Geometry check sheet. Reference: the model listing, model coordinates, mm. Face numbers are marked on the shaded views. A direction names the side the tool comes from. Coordinates: 2 decimals unless noted, no trailing zeros. Write each loop counter-clockwise with the first axis right and the second up, starting at its lowest first coordinate (ties: lowest second). Pieces come first, ordered by that corner, then holes.
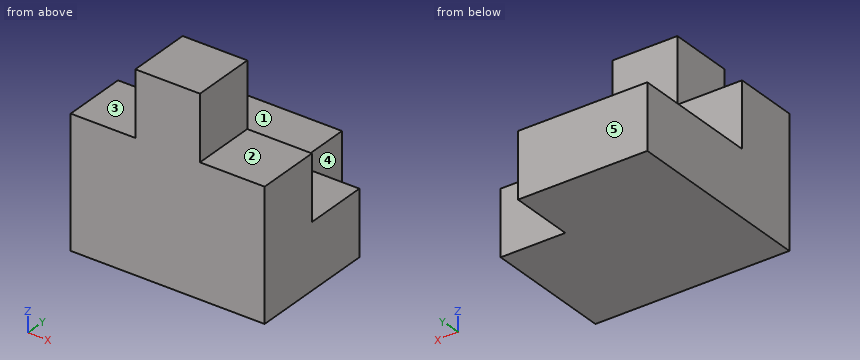
from build123d import *

# Parameters (mm, degrees)
ESBO_O2_W                = 60
ESBO_O2_H                = 20
RESSALTO_EXTRUS_O1_DEPTH = 40
ESBO_O4_W                = 20
ESBO_O4_H                = 20
CORTE_EXTRUS_O1_DEPTH    = 40
ESBO_O5_W                = 20
ESBO_O5_H                = 20
CORTE_EXTRUS_O2_DEPTH    = 40
ESBO_O7_W                = 60
ESBO_O7_H                = 40.049473908
RESSALTO_EXTRUS_O2_DEPTH = 20
ESBO_O8_W                = 40
ESBO_O8_H                = 20
RESSALTO_EXTRUS_O3_DEPTH = 20


with BuildPart() as part:
    # Esboço2 → Ressalto-extrusão1 (new body)
    with BuildSketch(Plane.XY):
        with Locations((30, 10)):
            Rectangle(ESBO_O2_W, ESBO_O2_H)
    extrude(amount=RESSALTO_EXTRUS_O1_DEPTH)

    # Esboço4 → Corte-extrusão1 (cut)
    with BuildSketch(Plane(origin=(0, 20, 0), x_dir=(1, 0, 0), z_dir=(0, 1, 0))):
        with Locations((10, -30)):
            Rectangle(ESBO_O4_W, ESBO_O4_H)
    extrude(amount=-CORTE_EXTRUS_O1_DEPTH, mode=Mode.SUBTRACT)

    # Esboço5 → Corte-extrusão2 (cut)
    with BuildSketch(Plane(origin=(0, 20, 0), x_dir=(1, 0, 0), z_dir=(0, 1, 0))):
        with Locations((50, -30)):
            Rectangle(ESBO_O5_W, ESBO_O5_H)
    extrude(amount=-CORTE_EXTRUS_O2_DEPTH, mode=Mode.SUBTRACT)

    # Esboço7 → Ressalto-extrusão2 (add)
    with BuildSketch(Plane(origin=(0, 0, 0), x_dir=(-1, 0, 0), z_dir=(0, 0, -1))):
        with Locations((-30, 20.024736954)):
            Rectangle(ESBO_O7_W, ESBO_O7_H)
    extrude(amount=RESSALTO_EXTRUS_O2_DEPTH)

    # Esboço8 → Ressalto-extrusão3 (add)
    with BuildSketch(Plane(origin=(0, 40.049473908, 0), x_dir=(1, 0, 0), z_dir=(0, 1, 0))):
        with Locations((20, 10)):
            Rectangle(ESBO_O8_W, ESBO_O8_H)
    extrude(amount=RESSALTO_EXTRUS_O3_DEPTH)


solid = part.part
1. Access from +Z, -Z, +X, -X, +Y, -Y to the whole of each face (thin tool, end or side, straight path). Record for the marked faces 1, 2, 3, 4 and 5.
Computed values:
face 1: +Z, +X, -X, +Y
face 2: +Z, +X, +Y, -Y
face 3: +Z, -X, +Y, -Y
face 4: +Z, -Z, +X, +Y
face 5: +Z, -Z, +X, -X, +Y
2. Gauge pin test, flat ends, axial feed: pin 1 Ø20 at (x, y) = (19.5, 30.5) entering from +Z; pin 2 Ø10 at (x, y) = (14.5, 15) entering from +Z; pin 3 Ø16 at (y, z) = (51.5, -14.5) entering from +X. Record the tip position at first contact, or that the pin passes through.
Computed values:
pin 1: stops at z = 0
pin 2: stops at z = 20
pin 3: stops at x = 40
3. Sectioned sample at B-B, the plane z = -1. Record the boundary of the cut face in (x, y).
Computed values:
outline: (0, 0) - (60, 0) - (60, 40.05) - (40, 40.05) - (40, 60.05) - (0, 60.05) - close
4. Sectioned sample at C-C, the plane x = 29. Record the boundary of the cut face in (y, z), and give its area (3 significant figures).
Computed values:
outline: (0, -20) - (60.05, -20) - (60.05, 0) - (20, 0) - (20, 40) - (0, 40) - close
area: 2,000 mm2
5. Thickness scan on line 1 along Y through (x, z) = (34, 17.5); line 2 along Z through (x, y) = (57.5, 11); line 3 along Y through (x, z) = (50, -10). Record the ranges inside material, lowest first.
Computed values:
line 1: y = 0 to 20
line 2: z = -20 to 20
line 3: y = 0 to 40.05
6. Sectioned sample at D-D, the plane z = 21. Record the boundary of the cut face in (x, y), and give its area (3 significant figures).
Computed values:
outline: (20, 0) - (40, 0) - (40, 20) - (20, 20) - close
area: 400 mm2
7. Sectioned sample at A-A, the plane y = 14. Record the boundary of the cut face in (x, z), and give its area (3 significant figures).
Computed values:
outline: (0, -20) - (60, -20) - (60, 20) - (40, 20) - (40, 40) - (20, 40) - (20, 20) - (0, 20) - close
area: 2,800 mm2
